Source: CAD feature listing. Evaluate the final solid. Frame: model axes, mm. A direction names the side the tool comes from. Round coordinates to 2 decimals unless told otherwise and drop trailing zeros. Loops run counter-clockwise (first coordinate to the right, second up) from the corner with the lowest first, then second, coordinate; pieces in that order, holes last.
(1) Set-up query: faces 1 (the cylindrical face through (73.986, -136.65, -138.127)), 2 (the flat face through (40.21, -106.21, -105.92)), 3 (the flat face through (70, -80, 1)). Return all of +Z, -Z, +X, -X, +Y, -Y with unobstructed straight access to the full face (end or side cutting, diameter ignored); none if empty.
(2) Section A-A, the plane x = 73. Return the cut outline in (y, z).
(3) Mould query, pull axis Y, two halves, no side actions, for faces 4 (the flat face through (40, 16, -200)), 5 (the flat face through (60, 1, 1)), 6 (the cylindrical face through (6.014, -138.127, 136.65)). Classes: pulls with the +Y half, pulls with the -Y half, needs draft (parallel to the pull), parting line crosses it, or undercut.
(4) Material intervals for probe 1 along Y at (x, z) = (59, -75); probe 2 along X at (y, z) = (0, 168); probe 3 along Y at (x, z) = (34, -73), sorted ascending.
(5) Section D-D, the plane x = 33. Count the separate pieces of the cut face and the enclosed holes in it, plus the area to 3 significant figures.
(6) Section B-B, the plane y = -51.5. Return the cut outline in (x, z).
(7) First-contact query: pin 1 Ø24 at (x, y) = (33, -6.5) entering from +Z; pin 2 Ø6 at (x, y) = (65, -20.5) entering from -Z; pin 3 Ø12 at (x, y) = (68, -45) entering from +Z; pin 4 Ø16 at (y, z) = (-100, 75) entering from -X. Flat tips, straight axial feed; report the tip coordinate or a pass-through.
(8) Section C-C, the plane y = 0. Return the cut outline in (x, z), plus the area to 3 significant figures.
```python
from build123d import *

# Parameters (mm, degrees)
BOSS_EXTRUDE2_DEPTH = 80
FILLET2_R           = 20
SKETCH5_R           = 15
CUT_EXTRUDE2_DEPTH  = 50
CIRPATTERN3_COUNT   = 8
SKETCH6_R           = 5
CUT_EXTRUDE3_DEPTH  = 294.938769134
SKETCH7_W           = 180
SKETCH7_H           = 160
CUT_EXTRUDE4_DEPTH  = 20
CHAMFER1_SIZE       = 10


with BuildPart() as part:
    # Sketch4 → Boss-Extrude2 (new body)
    with BuildSketch(Plane(origin=(0, 0, 0), x_dir=(0, 0, -1), z_dir=(1, 0, 0))):
        Polygon((82.842712475, 200), (-82.842712475, 200), (-200, 82.842712475), (-200, -82.842712475), (-82.842712475, -200), (82.842712475, -200), (200, -82.842712475), (200, 82.842712475), align=None)
    extrude(amount=BOSS_EXTRUDE2_DEPTH)

    # Fillet2
    fillet2_edges = [part.edges().sort_by_distance(p)[0] for p in [
        (80, 141.421356237, 141.421356237),
        (0, 200, 0),
        (0, 141.421356237, -141.421356237),
        (80, 0, 200),
        (40, 82.842712475, -200),
        (40, -82.842712475, -200),
        (40, -200, -82.842712475),
        (40, -200, 82.842712475),
        (40, -82.842712475, 200),
        (40, 82.842712475, 200),
        (40, 200, 82.842712475),
        (40, 200, -82.842712475),
        (80, -141.421356237, 141.421356237),
        (80, -200, 0),
        (80, -141.421356237, -141.421356237),
        (80, 0, -200),
        (80, 141.421356237, -141.421356237),
        (80, 200, 0),
        (0, 0, -200),
        (0, -141.421356237, -141.421356237),
        (0, -200, 0),
        (0, -141.421356237, 141.421356237),
        (0, 0, 200),
        (0, 141.421356237, 141.421356237),
    ]]
    fillet(fillet2_edges, radius=FILLET2_R)

    # Sketch5 → Cut-Extrude2 (cut)
    with BuildSketch(Plane(origin=(0, -141.421356237, -141.421356237), x_dir=(1, 0, 0), z_dir=(0, -0.7071067811865474, -0.7071067811865477))):
        with Locations(Location((40, 0, 0), (0, 0, 270))):
            Circle(SKETCH5_R)
    cut_extrude2 = extrude(amount=-CUT_EXTRUDE2_DEPTH, mode=Mode.SUBTRACT)

    # CirPattern3: Cut-Extrude2 ×8 about axis
    cirpattern3_axis = Axis((0, 0, 0), (1, 0, 0))
    for i in range(1, CIRPATTERN3_COUNT):
        add(cut_extrude2.rotate(cirpattern3_axis, i * 360 / CIRPATTERN3_COUNT), mode=Mode.SUBTRACT)

    # Sketch6 → Cut-Extrude3 (cut, through all)
    with BuildSketch(Plane.ZY):
        with Locations((75, 100)):
            Circle(SKETCH6_R)
        with Locations(Location((-75, 100, 0), (0, 0, 180))):
            Circle(SKETCH6_R)
        with Locations((-75, -100)):
            Circle(SKETCH6_R)
        with Locations(Location((75, -100, 0), (0, 0, 180))):
            Circle(SKETCH6_R)
    extrude(amount=-CUT_EXTRUDE3_DEPTH, mode=Mode.SUBTRACT)

    # Sketch7 → Cut-Extrude4 (cut)
    with BuildSketch(Plane(origin=(80, 0, 0), x_dir=(0, 0, -1), z_dir=(1, 0, 0))):
        Rectangle(SKETCH7_W, SKETCH7_H)
    extrude(amount=-CUT_EXTRUDE4_DEPTH, mode=Mode.SUBTRACT)

    # Chamfer1
    chamfer1_edges = [part.edges().sort_by_distance(p)[0] for p in [
        (0, -100, 80),
        (0, -100, -80),
        (0, 100, -70),
        (0, 100, 70),
    ]]
    chamfer(chamfer1_edges, length=CHAMFER1_SIZE)


solid = part.part
```
Output values:
1. face 1: -Z, +X, -Y
1. face 2: none
1. face 3: +X
2. outline: (-195.2, -74.56) arc R15.2 ccw to (-190.75, -85.31) - (-85.31, -190.75) arc R15.2 ccw to (-74.56, -195.2) - (74.56, -195.2) arc R15.2 ccw to (85.31, -190.75) - (190.75, -85.31) arc R15.2 ccw to (195.2, -74.56) - (195.2, 74.56) arc R15.2 ccw to (190.75, 85.31) - (85.31, 190.75) arc R15.2 ccw to (74.56, 195.2) - (-74.56, 195.2) arc R15.2 ccw to (-85.31, 190.75) - (-190.75, 85.31) arc R15.2 ccw to (-195.2, 74.56) - close; hole circle Ø10 at (-100, -75); hole circle Ø10 at (-100, 75); hole (-80, -90) - (80, -90) - (80, 90) - (-80, 90) - close; hole circle Ø10 at (100, -75); hole circle Ø10 at (100, 75)
3. face 4: needs draft
3. face 5: undercut
3. face 6: pulls with the -Y half
4. probe 1: y = -200 to -105, -95 to 95, 105 to 200
4. probe 2: x = 0 to 25, 55 to 80
4. probe 3: y = -200 to -104.58, -95.42 to 95.42, 104.58 to 200
5. separate pieces: 1
5. enclosed holes: 4
5. area: 122,000 mm2
6. outline: (0, -180) arc R20 ccw to (20, -200) - (60, -200) arc R20 ccw to (80, -180) - (80, -90) - (60, -90) - (60, 90) - (80, 90) - (80, 180) arc R20 ccw to (60, 200) - (20, 200) arc R20 ccw to (0, 180) - close
7. pin 1: stops at z = 200
7. pin 2: stops at z = -199.9
7. pin 3: stops at z = 199.9
7. pin 4: stops at x = 7
8. outline: (0, -180) arc R20 ccw to (20, -200) - (25, -200) - (25, -150) - (55, -150) - (55, -200) - (60, -200) arc R20 ccw to (80, -180) - (80, -90) - (60, -90) - (60, 90) - (80, 90) - (80, 180) arc R20 ccw to (60, 200) - (55, 200) - (55, 150) - (25, 150) - (25, 200) - (20, 200) arc R20 ccw to (0, 180) - close
8. area: 25,100 mm2
